from build123d import *

# Parameters (mm, degrees)
SKETCH1_W                                       = 89
SKETCH1_H                                       = 23.2
BOSS_EXTRUDE1_DEPTH                             = 4
BOSS_EXTRUDE1_DEPTH_BACK                        = 1.9
M2_5X0_45_TAPPED_HOLE2_D                        = 2.05
M2_5X0_45_TAPPED_HOLE2_CSINK_D                  = 2.55
M2_5X0_45_TAPPED_HOLE2_CSINK_ANGLE              = 90
CSK_FOR_M2_FLAT_HEAD_MACHINE_SCREW1_D           = 2.4
CSK_FOR_M2_FLAT_HEAD_MACHINE_SCREW1_DEPTH       = 6.45
CSK_FOR_M2_FLAT_HEAD_MACHINE_SCREW1_CSINK_D     = 4.4
CSK_FOR_M2_FLAT_HEAD_MACHINE_SCREW1_CSINK_ANGLE = 90
CSK_FOR_M2_FLAT_HEAD_MACHINE_SCREW1_TIP         = 0.721032743
CUT_EXTRUDE1_DEPTH                              = 23.2


with BuildPart() as part:
    # Sketch1 → Boss-Extrude1 (new body, two sides)
    with BuildSketch(Plane(origin=(0, 0, 0), x_dir=(1, 0, 0), z_dir=(0, 1, 0))) as boss_extrude1_sk:
        Rectangle(SKETCH1_W, SKETCH1_H)
    extrude(amount=BOSS_EXTRUDE1_DEPTH)
    extrude(boss_extrude1_sk.sketch, amount=-BOSS_EXTRUDE1_DEPTH_BACK)

    # M2.5x0.45 Tapped Hole2 (through all)
    with Locations(Plane(origin=(0, 4, 0), x_dir=(1, 0, 0), z_dir=(0, 1, 0))):
        with Locations((-22, 6.6), (-22, -1.4), (22, -1.4), (22, 6.6), (0, 2.6)):
            CounterSinkHole(M2_5X0_45_TAPPED_HOLE2_D / 2, M2_5X0_45_TAPPED_HOLE2_CSINK_D / 2, counter_sink_angle=M2_5X0_45_TAPPED_HOLE2_CSINK_ANGLE)

    # CSK for M2 Flat Head Machine Screw1
    with Locations(Plane(origin=(0, 4, 0), x_dir=(1, 0, 0), z_dir=(0, 1, 0))):
        with Locations((-36.5, -1.1), (-39.5, -9.1), (-30, -9.1), (30, -9.1), (39.5, -9.1), (36.5, -1.1)):
            CounterSinkHole(CSK_FOR_M2_FLAT_HEAD_MACHINE_SCREW1_D / 2, CSK_FOR_M2_FLAT_HEAD_MACHINE_SCREW1_CSINK_D / 2, depth=CSK_FOR_M2_FLAT_HEAD_MACHINE_SCREW1_DEPTH, counter_sink_angle=CSK_FOR_M2_FLAT_HEAD_MACHINE_SCREW1_CSINK_ANGLE)
            with Locations((0, 0, -(CSK_FOR_M2_FLAT_HEAD_MACHINE_SCREW1_DEPTH + CSK_FOR_M2_FLAT_HEAD_MACHINE_SCREW1_TIP / 2))):  # 118° drill point
                Cone(0, CSK_FOR_M2_FLAT_HEAD_MACHINE_SCREW1_D / 2, CSK_FOR_M2_FLAT_HEAD_MACHINE_SCREW1_TIP, mode=Mode.SUBTRACT)

    # Sketch8 → Cut-Extrude1 (cut)
    with BuildSketch(Plane.XY.offset(11.6)):
        Polygon((41.5, 4), (44.5, 4), (44.5, 1), align=None)
        Polygon((-44.5, 4), (-44.5, 1), (-41.5, 4), align=None)
    extrude(amount=-CUT_EXTRUDE1_DEPTH, mode=Mode.SUBTRACT)


solid = part.part
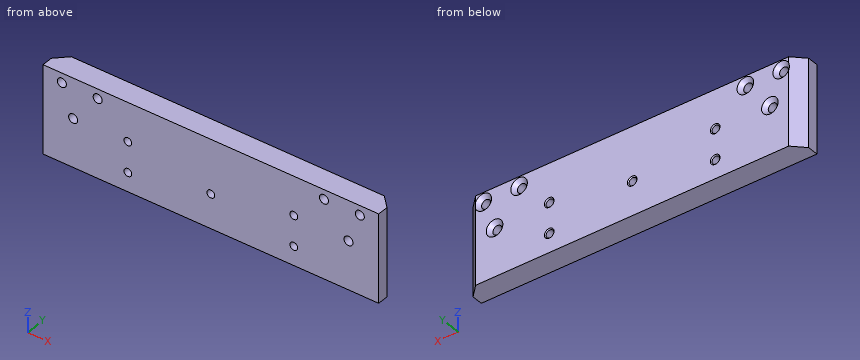
Input: part model. Units: mm. Frame: model coordinates. Coordinates: 2 decimals unless noted, no trailing zeros. Loops run counter-clockwise (first coordinate to the right, second up) from the corner with the lowest first, then second, coordinate; pieces in that order, holes last. Notation, with made-up numbers: (-17.75, -15) - (-5.75, -15) arc R19 cw to (-5.75, 3) - close; hole circle Ø8 at (86.5, 19). An arc over 180 degrees is marked (long way). Answer in a Markdown table with one row per item. Add a question column.
Item 1: Section query B-B on z = -2.6. Return the cut outline in (x, y) (3 decimals), then the cut area to 3 significant figures.
Item 2: Section query A-A on x = 22. Return the cut outline in (y, z) (3 decimals), then the cut area to 3 significant figures.
Item 3: Section query D-D on x = 0. Return the cut outline in (y, z) (3 decimals).
Item 4: Section query C-C on z = 9.1. Return the cut outline in (x, y), then the cut area to 3 significant figures.
Item 5: Contact query for flat-ended pins moving along their axis: P1, Ø1.8, axis at x = -22, z = -6.6, coming from the +Y side; P2, Ø3, axis at x = -39.5, z = 9.1, coming from the +Y side; P3, Ø3.5, axis at x = 22, z = 1.4, coming from the -Y side. Output: stop coordinate, or through.
Item 6: Line query: line 1 along Z through (x, y) = (22, -0.6) (3 decimals); line 2 along X through (y, z) = (0.7, -6.6) (3 decimals); line 3 along Z through (x, y) = (30, -0.1). Output: solid intervals per line, ascending. Write a range as [from, to].
Recorded:
| question | item | result |
|---|---|---|
| 1 | outline | (-44.5, -1.9) - (-1.025, -1.9) - (-1.025, 3.75) - (-1.275, 4) - (-41.5, 4) - (-44.5, 1) - close; (1.025, -1.9) - (44.5, -1.9) - (44.5, 1) - (41.5, 4) - (1.275, 4) - (1.025, 3.75) - close |
| 1 | area | 504 mm^2 |
| 2 | outline | (-1.9, -11.6) - (4, -11.6) - (4, -7.875) - (3.75, -7.625) - (-1.9, -7.625) - close; (-1.9, -5.575) - (3.75, -5.575) - (4, -5.325) - (4, 0.125) - (3.75, 0.375) - (-1.9, 0.375) - close; (-1.9, 2.425) - (3.75, 2.425) - (4, 2.675) - (4, 11.6) - (-1.9, 11.6) - close |
| 2 | area | 113 mm^2 |
| 3 | outline | (-1.9, -11.6) - (4, -11.6) - (4, -3.875) - (3.75, -3.625) - (-1.9, -3.625) - close; (-1.9, -1.575) - (3.75, -1.575) - (4, -1.325) - (4, 11.6) - (-1.9, 11.6) - close |
| 4 | outline | (-44.5, -1.9) - (-40.7, -1.9) - (-40.7, 3) - (-41.6, 3.9) - (-44.5, 1) - close; (-38.3, -1.9) - (-31.2, -1.9) - (-31.2, 3) - (-32.2, 4) - (-37.3, 4) - (-38.3, 3) - close; (-28.8, -1.9) - (28.8, -1.9) - (28.8, 3) - (27.8, 4) - (-27.8, 4) - (-28.8, 3) - close; (31.2, -1.9) - (38.3, -1.9) - (38.3, 3) - (37.3, 4) - (32.2, 4) - (31.2, 3) - close; (40.7, -1.9) - (44.5, -1.9) - (44.5, 1) - (41.6, 3.9) - (40.7, 3) - close |
| 4 | area | 455 mm^2 |
| 5 | P1 | through |
| 5 | P2 | y = 3.3 |
| 5 | P3 | y = -1.9 |
| 6 | line 1 | [-11.6, -7.625], [-5.575, 0.375], [2.425, 11.6] |
| 6 | line 2 | [-44.5, -23.025], [-20.975, 20.975], [23.025, 44.5] |
| 6 | line 3 | [-11.6, 7.9], [10.3, 11.6] |
